Check sheet for the modelled part. Datum: model origin and axes. Units: mm. Face numbers are marked on the shaded views. A direction names the side the tool comes from. Round coordinates to 2 decimals unless told otherwise and drop trailing zeros. Loops run counter-clockwise (first coordinate to the right, second up) from the corner with the lowest first, then second, coordinate; pieces in that order, holes last. Notation, with made-up numbers: (69, 29.5) -> (95, 29.5) arc R22 cw to (95, 61.5) -> close; hole circle Ø10 at (-35, 10). An arc over 180 degrees is marked (long way). One line per item, written item: value. Start each with the question number.
1. Cross-section at D-D on z = 30. Record the cut outline in (x, y), then the cut area to 3 significant figures.
2. Set-up check for the marked faces 4, 5, 6, 7 and 8: record each of +Z, -Z, +X, -X, +Y, -Y from which the full face is reachable in a straight line by a thin tool's end or side.
3. Release check for a two-part mould opening along Y. For the marked faces 1, 2 and 3 record: +Y half, -Y half, draft (parallel to the pull), parting line (faces both ways), or undercut.
4. Material ranges on L1, parallel to X at y = 11.25, z = 5; L2, parallel to Y at x = -11.25, z = 43; L3, parallel to Z at x = -13, y = 0, recorded low to high.
5. Go/stop test with flat-tipped pins: pin 1 (1.2 mm diameter, centred on y = 0, z = 33, fed in from +X); pin 2 (5 mm diameter, centred on x = -3, z = -4, fed in from -Y); pin 3 (0.6 mm diameter, centred on x = -0.5, z = 43, fed in from +Y). Record where each tip stops, or that it passes through.
6. Cross-section at A-A on x = 12. Count the separate pieces of the cut face and the enclosed holes in it, then the cut area to 3 significant figures.
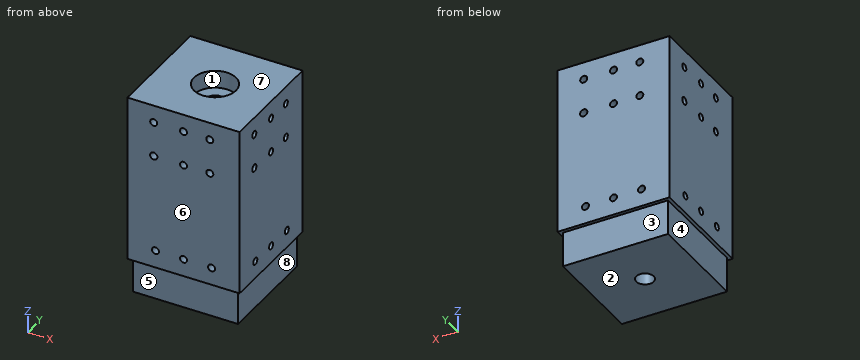
Autodesk Inventor part; units mm, degrees
ref_plane "YZ Plane" through (0, 0, 0) normal (1, 0, 0) x (0, 1, 0)
ref_plane "XZ Plane" through (0, 0, 0) normal (0, 1, 0) x (-1, 0, 0)
ref_plane "XY Plane" through (0, 0, 0) normal (0, 0, 1) x (1, 0, 0)
sketch "Skizze1" plane through (0, 0, 0) normal (0, 0, 1) x (1, 0, 0)
  line L0 (-16, 16) -> (16, 16)
  line L1 (16, 16) -> (16, -16)
  line L2 (16, -16) -> (-16, -16)
  line L3 (-16, -16) -> (-16, 16)
  line L4 (-16, 16) -> (16, -16) construction
  line L5 (16, 16) -> (-16, -16) construction
  point P0 (0, 0)
  dimension "d0" = 32
  dimension "d1" = 32
extrude "Extrusion1" add sketch "Skizze1" along normal blind 48
sketch "Skizze2" plane through (-16, 16, 0) normal (0, 1, 0) x (1, 0, 0)
  line L0 (0, 0) -> (32, 0) construction
  line L1 (0, 0) -> (0, -48) construction
  line L2 (32, -48) -> (0, -48) construction
  line L3 (32, 0) -> (32, -48) construction
  line L4 (5, -43) -> (5, -5)
  line L5 (5, -5) -> (27, -5)
  line L6 (27, -5) -> (27, -43)
  line L7 (27, -43) -> (5, -43)
  line L8 (32, -48) -> (0, -48)
  line L9 (16, -48) -> (16, 0)
  circle A0 centre (16, -5) radius 1
  circle A1 centre (8, -5) radius 1
  circle A2 centre (24, -5) radius 1
  circle A3 centre (16, -43) radius 1
  circle A4 centre (8.5, -43) radius 1
  circle A5 centre (24.5, -43) radius 1
  line L10 (27, -33) -> (5, -33)
  circle A6 centre (24.5, -33) radius 1.0474
  circle A7 centre (16, -33) radius 1
  circle A8 centre (8.5, -33) radius 1
  dimension "d4" = 5
  dimension "d5" = 2
  dimension "d6" = 2
  dimension "d7" = 2
  dimension "d8" = 2
  dimension "d9" = 8
  dimension "d10" = 8
  dimension "d11" = 2
  dimension "d12" = 2
  dimension "d23" = 10
extrude "Extrusion2" cut sketch "Skizze2" against normal blind 8 contours A4 L7 | L7 A4 | A8 L10 | L10 A8 | A1 L5 | L5 A1 | A3 L9 L7 | L7 L9 A3 | A7 L9 L10 | L10 L9 A7 | L9 A3 L7 | L7 A3 L9 | A0 L9 L5 | L5 L9 A0 | L10 A7 L9 | L9 A7 L10 | L9 A0 L5 | L5 A0 L9 | A5 L7 | L7 A5 | A6 L10 | L10 A6 | A2 L5 | L5 A2
sketch "Skizze3" plane through (0, 0, 48) normal (0, 0, 1) x (1, 0, 0)
  circle A0 centre (0, 0) radius 2.5
  dimension "d15" = 5
extrude "Extrusion3" cut sketch "Skizze3" against normal through all
sketch "Skizze4" plane through (0, 0, 48) normal (0, 0, 1) x (1, 0, 0)
  line L0 (-2.45, 0.55) -> (-42.45, 0.55)
  circle A0 centre (0, 0) radius 2.5
  line L1 (16, 16) -> (-16, 16)
  line L2 (-16, 16) -> (-16, -16)
  line L3 (-16, -16) -> (16, -16)
  line L4 (16, -16) -> (16, 16)
  circle A1 centre (0, 0) radius 6
  dimension "d18" = 12
extrude "Extrusion4" cut sketch "Skizze4" against normal blind 5 contours A1
sketch "Skizze5" plane through (0, 0, 0) normal (0, 0, -1) x (-1, 0, 0)
  line L0 (-15, -15) -> (15, -15)
  line L1 (15, -15) -> (15, 15)
  line L2 (15, 15) -> (-15, 15)
  line L3 (-15, 15) -> (-15, -15)
  circle A0 centre (0, 0) radius 2.5
  line L4 (-15, -15) -> (15, 15) construction
  line L5 (15, -15) -> (-15, 15) construction
  dimension "d24" = 30
  dimension "d25" = 30
extrude "Extrusion5" add sketch "Skizze5" along normal blind 10
pattern_circular "Runde Anordnung1" count 4 over 360 about axis through (0, 0, 48) along (0, 0, -1) of "Extrusion2"
properties part number "LASER_640nm"
Taken from the geometry:
1. outline: (-16, -16) -> (16, -16) -> (16, 16) -> (-16, 16) -> close; hole circle Ø5 at (0, 0)
1. area: 1,000 mm2
2. face 4: -Z, -X, +Y, -Y
2. face 5: -Z, +X, -X, -Y
2. face 6: +Z, -Z, +X, -X, -Y
2. face 7: +Z, +X, -X, +Y, -Y
2. face 8: -Z, +X, +Y, -Y
3. face 1: undercut
3. face 2: draft
3. face 3: +Y half
4. L1: x = -16 to -9, -7 to -1, 1 to 7, 9 to 16
4. L2: y = -16 to -8.5, -6.5 to -1, 1 to 7.5, 9.5 to 16
4. L3: z = -10 to 4, 6 to 32, 34 to 42, 44 to 48
5. pin 1: stops at x = 8
5. pin 2: stops at y = -15
5. pin 3: stops at y = 8
6. separate pieces: 1
6. enclosed holes: 9
6. area: 1,810 mm2
